Verification items for the finished model (mm, model axes). Face numbers are marked on the shaded views. A direction names the side the tool comes from. Coordinates: 2 decimals unless noted, no trailing zeros. Write each loop counter-clockwise with the first axis right and the second up, starting at its lowest first coordinate (ties: lowest second). Pieces come first, ordered by that corner, then holes.
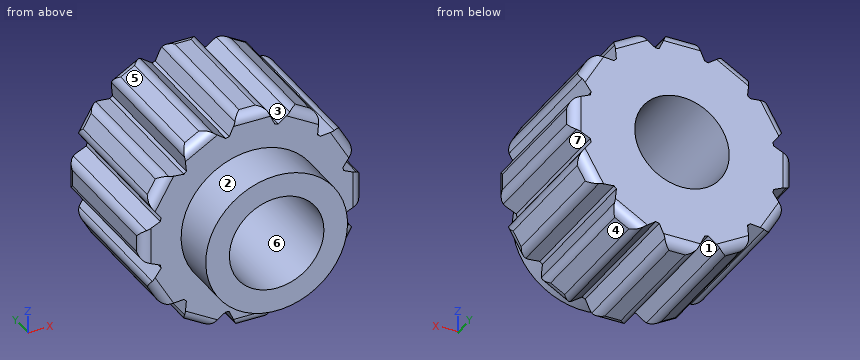
```python
from build123d import *

# Parameters (mm, degrees)
SKETCH1_R           = 12.7
BOSS_EXTRUDE1_DEPTH = 19.05
BOSS_EXTRUDE2_DEPTH = 19.05
CIRPATTERN1_COUNT   = 12
FILLET1_R           = 1.27
SKETCH3_R           = 9.525
BOSS_EXTRUDE3_DEPTH = 6.35
SKETCH4_R           = 6.35
CUT_EXTRUDE1_DEPTH  = 33.965736182


with BuildPart() as part:
    # Sketch1 → Boss-Extrude1 (new body)
    with BuildSketch(Plane(origin=(0, 0, 0), x_dir=(1, 0, 0), z_dir=(0, 1, 0))):
        with Locations(Location((0, 0, 0), (0, 0, 90))):
            Circle(SKETCH1_R)
    extrude(amount=BOSS_EXTRUDE1_DEPTH)

    # Sketch2 → Boss-Extrude2 (add)
    with BuildSketch(Plane(origin=(0, 19.05, 0), x_dir=(1, 0, 0), z_dir=(0, 1, 0))):
        Polygon((-1.905, 14.859), (1.905, 14.859), (3.368404775, 11.639782335), (-3.368404775, 11.639782335), align=None)
    boss_extrude2 = extrude(amount=-BOSS_EXTRUDE2_DEPTH)

    # CirPattern1: Boss-Extrude2 ×12 about axis
    cirpattern1_axis = Axis((0, 0, 0), (0, 1, 0))
    for i in range(1, CIRPATTERN1_COUNT):
        add(boss_extrude2.rotate(cirpattern1_axis, i * 360 / CIRPATTERN1_COUNT))

    # Fillet1
    fillet1_edges = [part.edges().sort_by_distance(p)[0] for p in [
        (0, 19.05, -14.859),
        (1.905, 9.525, -14.859),
        (-12.868271475, 0, -7.4295),
        (-13.820771475, 9.525, -5.779721606),
        (-14.859, 0, 0),
        (-14.859, 9.525, 1.905),
        (-12.868271475, 0, 7.4295),
        (-11.915771475, 9.525, 9.079278394),
        (-7.4295, 0, 12.868271475),
        (-5.779721606, 9.525, 13.820771475),
        (0, 0, 14.859),
        (1.905, 9.525, 14.859),
        (7.4295, 0, 12.868271475),
        (9.079278394, 9.525, 11.915771475),
        (12.868271475, 0, 7.4295),
        (13.820771475, 9.525, 5.779721606),
        (14.859, 0, 0),
        (14.859, 9.525, -1.905),
        (12.868271475, 0, -7.4295),
        (11.915771475, 9.525, -9.079278394),
        (0, 0, -14.859),
        (7.4295, 0, -12.868271475),
        (5.779721606, 9.525, -13.820771475),
        (-1.905, 9.525, -14.859),
        (7.4295, 19.05, -12.868271475),
        (12.868271475, 19.05, -7.4295),
        (14.859, 19.05, 0),
        (12.868271475, 19.05, 7.4295),
        (7.4295, 19.05, 12.868271475),
        (0, 19.05, 14.859),
        (-7.4295, 19.05, 12.868271475),
        (-12.868271475, 19.05, 7.4295),
        (-14.859, 19.05, 0),
        (-12.868271475, 19.05, -7.4295),
        (-7.4295, 19.05, -12.868271475),
        (-5.779721606, 9.525, -13.820771475),
        (-11.915771475, 9.525, -9.079278394),
        (-14.859, 9.525, -1.905),
        (-13.820771475, 9.525, 5.779721606),
        (-9.079278394, 9.525, 11.915771475),
        (-1.905, 9.525, 14.859),
        (5.779721606, 9.525, 13.820771475),
        (11.915771475, 9.525, 9.079278394),
        (14.859, 9.525, 1.905),
        (13.820771475, 9.525, -5.779721606),
        (9.079278394, 9.525, -11.915771475),
        (-7.4295, 0, -12.868271475),
        (-9.079278394, 9.525, -11.915771475),
    ]]
    fillet(fillet1_edges, radius=FILLET1_R)

    # Sketch3 → Boss-Extrude3 (add)
    with BuildSketch(Plane.XZ):
        with Locations(Location((0, 0, 0), (0, 0, 90))):
            Circle(SKETCH3_R)
    extrude(amount=BOSS_EXTRUDE3_DEPTH)

    # Sketch4 → Cut-Extrude1 (cut, through all)
    with BuildSketch(Plane.XZ.offset(6.35)):
        with Locations(Location((0, 0, 0), (0, 0, 270))):
            Circle(SKETCH4_R)
    extrude(amount=-CUT_EXTRUDE1_DEPTH, mode=Mode.SUBTRACT)


solid = part.part
```
1. Sectioned sample at B-B, the plane z = 0. Record the boundary of the cut face in (x, y) (3 decimals), and give its area (3 significant figures).
2. Sectioned sample at A-A, the plane x = 0. Record the boundary of the cut face in (y, z) (3 decimals), and give its area (3 significant figures).
3. Gauge pin test, flat ends, axial feed: P1, Ø5, axis at y = 8, z = -2, coming from the -X side; P2, Ø6, axis at x = 7.5, y = 7, coming from the +Z side; P3, Ø4, axis at x = 10.5, y = 12, coming from the -Z side; P4, Ø1, axis at y = 15, z = 11, coming from the -X side. Record the tip position at first contact, or that the pin passes through.
4. Draft check along Z on the marked faces 4, 5, 6 and 7. Enter one of: pulls with the +Z half, pulls with the -Z half, needs draft (parallel to the pull), parting line crosses it, or undercut.
5. Tool access check on the marked faces 1, 2 and 3. Record the directions out of +Z, -Z, +X, -X, +Y, -Y that give a thin tool (end or side, any length) a straight path to the whole face; none if there is none.
6. Sectioned sample at C-C, the plane y = -4. Record the boundary of the cut face in (x, z) (3 decimals), and give its area (3 significant figures).
7. Material ranges on L1, parallel to X at y = 12.5, z = 0; L2, parallel to X at y = -0.5, z = 0 (3 decimals); L3, parallel to X at y = 5, z = -6.5, recorded low to high.
Outcome:
1. outline: (-14.859, 1.27) arc R1.27 ccw to (-13.589, 0) - (-9.525, 0) - (-9.525, -6.35) - (-6.35, -6.35) - (-6.35, 19.05) - (-13.589, 19.05) arc R1.27 ccw to (-14.859, 17.78) - close; (6.35, -6.35) - (9.525, -6.35) - (9.525, 0) - (13.589, 0) arc R1.27 ccw to (14.859, 1.27) - (14.859, 17.78) arc R1.27 ccw to (13.589, 19.05) - (6.35, 19.05) - close
1. area: 363 mm2
2. outline: (-6.35, -9.525) - (0, -9.525) - (0, -13.589) arc R1.27 ccw to (1.27, -14.859) - (17.78, -14.859) arc R1.27 ccw to (19.05, -13.589) - (19.05, -6.35) - (-6.35, -6.35) - close; (-6.35, 6.35) - (19.05, 6.35) - (19.05, 13.589) arc R1.27 ccw to (17.78, 14.859) - (1.27, 14.859) arc R1.27 ccw to (0, 13.589) - (0, 9.525) - (-6.35, 9.525) - close
2. area: 363 mm2
3. P1: stops at x = -14.86
3. P2: stops at z = 13.58
3. P3: stops at z = -12.24
3. P4: stops at x = -9.01
4. face 4: pulls with the -Z half
4. face 5: pulls with the +Z half
4. face 6: undercut
4. face 7: undercut
5. face 1: -Z, +Y, -Y
5. face 2: -Y
5. face 3: +Z, +Y, -Y
6. outline: circle Ø19.05 at (0, 0); hole circle Ø12.7 at (0, 0)
6. area: 158 mm2
7. L1: x = -14.86 to -6.35, 6.35 to 14.86
7. L2: x = -9.525 to -6.35, 6.35 to 9.525
7. L3: x = -13.4 to 13.4
